from build123d import *

# Parameters (mm, degrees)
F1_DEPTH = 10
F2_W     = 12.5
F2_H     = 12.5
F3_DEPTH = 30
F5_D     = 3.175


with BuildPart() as f1:
    # F0 (on Front) → F1 (new body, symmetric)
    with BuildSketch(Plane.XZ):
        with BuildLine():
            Line((47.757359, 10), (0, 10))
            Line((0, 10), (0, -10))
            Line((0, -10), (33.757359, -10))
            ThreePointArc((33.757359, -10), (34.90541, -9.771639), (35.87868, -9.12132))
            Line((35.87868, -9.12132), (49.87868, 4.87868))
            ThreePointArc((49.87868, 4.87868), (50.528998, 8.14805), (47.757359, 10))
        make_face()
    extrude(amount=F1_DEPTH, both=True)

    # F2 (on face) → F3 (cut)
    with BuildSketch(Plane(origin=(0, 0, 0), x_dir=(0, -1, 0), z_dir=(-1, 0, 0))):
        Rectangle(F2_W, F2_H)
    extrude(amount=-F3_DEPTH, mode=Mode.SUBTRACT)

    # F5 (through all)
    with Locations(Plane.XZ.offset(10)):
        with Locations((6.2, 0)):
            Hole(F5_D / 2)


solid = f1.part
Can you work these out from the model? Positions are in its coordinate system, mm. A direction names the side the tool comes from. Coordinates: 2 decimals unless noted, no trailing zeros. Write each loop counter-clockwise with the first axis right and the second up, starting at its lowest first coordinate (ties: lowest second). Pieces come first, ordered by that corner, then holes.
Q1. Imagine slicing it at C-C, the plane y = -7.25. List the corners of the cut face in (x, z) for me (1 decimal).
Results found:
outline: (0, -10) - (33.8, -10) arc R3 ccw to (35.9, -9.1) - (49.9, 4.9) arc R3 ccw to (47.8, 10) - (0, 10) - close; hole circle Ø3.2 at (6.2, 0)
Q2. For P1, Ø2, axis at y = -3.5, z = -2.5, coming from the -X side, with a flat end and sliding along its axis, tell me the tip position at first contact or that it passes through.
Results found:
P1: stops at x = 30
Q3. Which directions (+Z, -Z, +X, -X, +Y, -Y) give clear straight access to the entire face, cutting with the end or side of a thin tool? Please do faces 1 (the face through (0, -7, 0)), 2 (the face through (15, 0, -6.25)).
Results found:
face 1: +Z, -Z, -X, +Y, -Y
face 2: -X
Q4. Imagine slicing it at A-A, the plane z = 0. List the corners of the cut face in (x, y) for me.
Results found:
outline: (0, -10) - (4.61, -10) - (4.61, -6.25) - (0, -6.25) - close; (0, 6.25) - (4.61, 6.25) - (4.61, 10) - (0, 10) - close; (7.79, -10) - (45, -10) - (45, 10) - (7.79, 10) - (7.79, 6.25) - (30, 6.25) - (30, -6.25) - (7.79, -6.25) - close
Q5. Please list where these lines run through material, in increasing order: L1, parallel to Z at x = 17, y = -5; L2, parallel to Z at x = 6.2, y = 7.9.
Results found:
L1: z = -10 to -6.25, 6.25 to 10
L2: z = -10 to -1.59, 1.59 to 10
Q6. If we mould it in two halves opening along X, with no side actions, what happens to faces 3 (the face through (17, 0, -10)), 4 (the face through (7.786, -8.099, 0.07)), 5 (the face through (7.786, 8.151, 0.07)), 6 (the face through (30, 0, 0))? For each: +X half, -X half, draft (parallel to the pull), parting line (faces both ways), or undercut.
Results found:
face 3: draft
face 4: undercut
face 5: undercut
face 6: -X half
Q7. Imagine slicing it at D-D, the plane x = 28. List the corners of the cut face in (y, z) for me.
Results found:
outline: (-10, -10) - (10, -10) - (10, 10) - (-10, 10) - close; hole (-6.25, -6.25) - (6.25, -6.25) - (6.25, 6.25) - (-6.25, 6.25) - close
Q8. Imagine slicing it at B-B, the plane x = 6.2. List the corners of the cut face in (y, z) for me.
Results found:
outline: (-10, -10) - (10, -10) - (10, -1.59) - (6.25, -1.59) - (6.25, -6.25) - (-6.25, -6.25) - (-6.25, -1.59) - (-10, -1.59) - close; (-10, 1.59) - (-6.25, 1.59) - (-6.25, 6.25) - (6.25, 6.25) - (6.25, 1.59) - (10, 1.59) - (10, 10) - (-10, 10) - close
